For this review, use the dimensioned drawing (mm, ordinates from the lowest corner) and the shaded views. A direction names the side the tool comes from. Give positions to 0.01 mm unless a question says otherwise; leave off trailing zeros. Loops run counter-clockwise (first coordinate to the right, second up) from the corner with the lowest first, then second, coordinate; pieces in that order, holes last. Notation, with made-up numbers: (29.5, 79.25) -> (78.5, 79.25) arc R30 ccw to (78.5, 112.25) -> close; hole circle Ø11 at (-26, -14.5). An arc over 180 degrees is marked (long way). Use a Markdown table: item, result. Add a question column.
1. Add section D-D (z = 0.5). State the section outline as (x, y) points, and give its area (3 significant figures).
2. Add section C-C (x = 23.75). State the section outline as (y, z) points, and give its area (3 significant figures).
3. For the marked faces 4, 5 and 6, list the 3-axis set-ups (+Z, -Z, +X, -X, +Y, -Y) from which the entire face can be reached by the end or side of a thin tool; tool diameter is ignored.
4. Add section B-B (x = 12). State the section outline as (y, z) points.
5. For pin 1 Ø4.5 at (x, y) = (12, 11) entering from -Z; pin 2 Ø2 at (x, z) = (2.5, 2) entering from +Y; pin 3 Ø4 at (y, z) = (14.5, 1.5) entering from -X; pin 4 Ø1.5 at (x, z) = (13, 4.5) entering from +Y, all flat-tipped, find the tip position at first contact; note any pin that passes through.
6. Add section A-A (z = 5.25). State the section outline as (x, y) points.
7. Draft analysis for pull direction X (two halves, no side actions). For the marked faces 1, 2 and 3, state which applies: pulls with the +X half, pulls with the -X half, needs draft (parallel to the pull), parting line crosses it, or undercut.
8. To check wall thickness, follow line 1 (Y direction, x = 12, z = 1.9); line 2 (Y direction, x = 24, z = 3); line 3 (Y direction, x = 22.5, z = 4.25). State the ranges of each line that lie inside material, in increasing order.
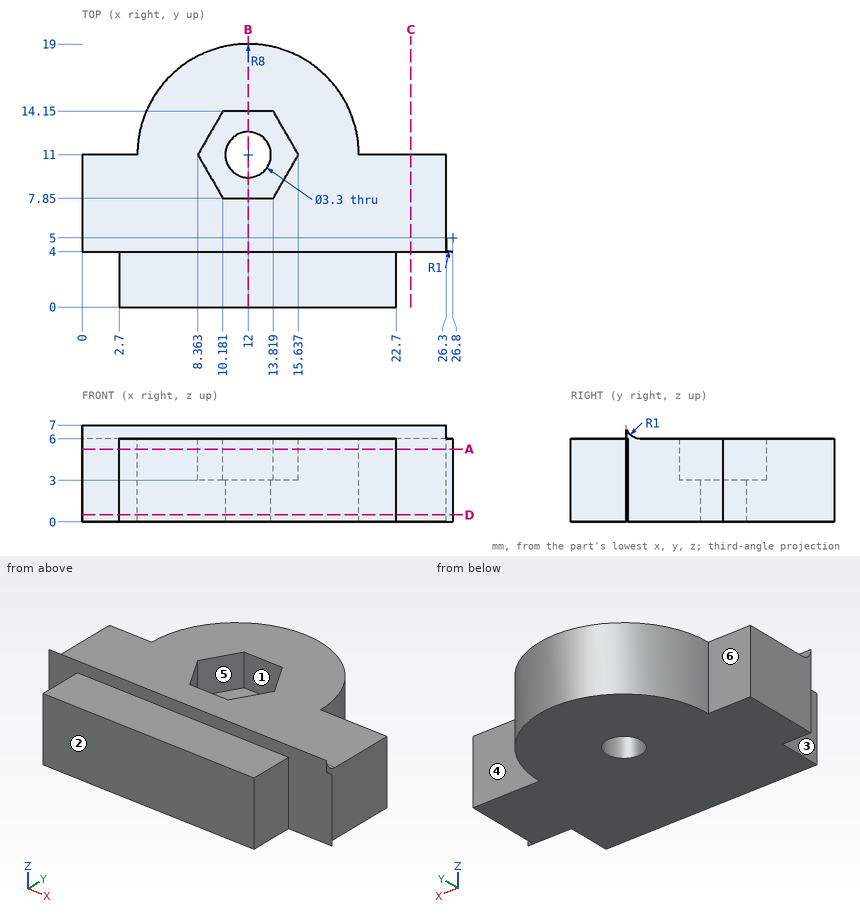
Taken from the geometry:
| question | item | result |
|---|---|---|
| 1 | outline | (0, 4) -> (2.7, 4) -> (2.7, 0) -> (22.7, 0) -> (22.7, 4) -> (26.8, 4) arc R1 cw to (26.3, 4.13) -> (26.3, 11) -> (20, 11) arc R8 ccw to (4, 11) -> (0, 11) -> close; hole circle Ø3.3 at (12, 11) |
| 1 | area | 356 mm^2 |
| 2 | outline | (4, 0) -> (11, 0) -> (11, 6) -> (5, 6) arc R1 cw to (4, 7) -> close |
| 2 | area | 42.2 mm^2 |
| 3 | face 4 | +Z, -Z, +X, +Y |
| 3 | face 5 | +Z |
| 3 | face 6 | +Z, -Z, -X, +Y |
| 4 | outline | (0, 0) -> (9.35, 0) -> (9.35, 3) -> (7.85, 3) -> (7.85, 6) -> (5, 6) arc R1 cw to (4, 7) -> (4, 6) -> (0, 6) -> close; (12.65, 0) -> (19, 0) -> (19, 6) -> (14.15, 6) -> (14.15, 3) -> (12.65, 3) -> close |
| 5 | pin 1 | stops at z = 0 |
| 5 | pin 2 | stops at y = 11 |
| 5 | pin 3 | stops at x = 4.14 |
| 5 | pin 4 | stops at y = 19 |
| 6 | outline | (0, 4) -> (2.7, 4) -> (2.7, 0) -> (22.7, 0) -> (22.7, 4) -> (26.8, 4) arc R1 cw to (26.3, 4.13) -> (26.3, 11) -> (20, 11) arc R8 ccw to (4, 11) -> (0, 11) -> close; hole (8.36, 11) -> (10.18, 7.85) -> (13.82, 7.85) -> (15.64, 11) -> (13.82, 14.15) -> (10.18, 14.15) -> close |
| 7 | face 1 | undercut |
| 7 | face 2 | needs draft |
| 7 | face 3 | pulls with the -X half |
| 8 | line 1 | y = 0 to 9.35, 12.65 to 19 |
| 8 | line 2 | y = 4 to 11 |
| 8 | line 3 | y = 0 to 11 |
